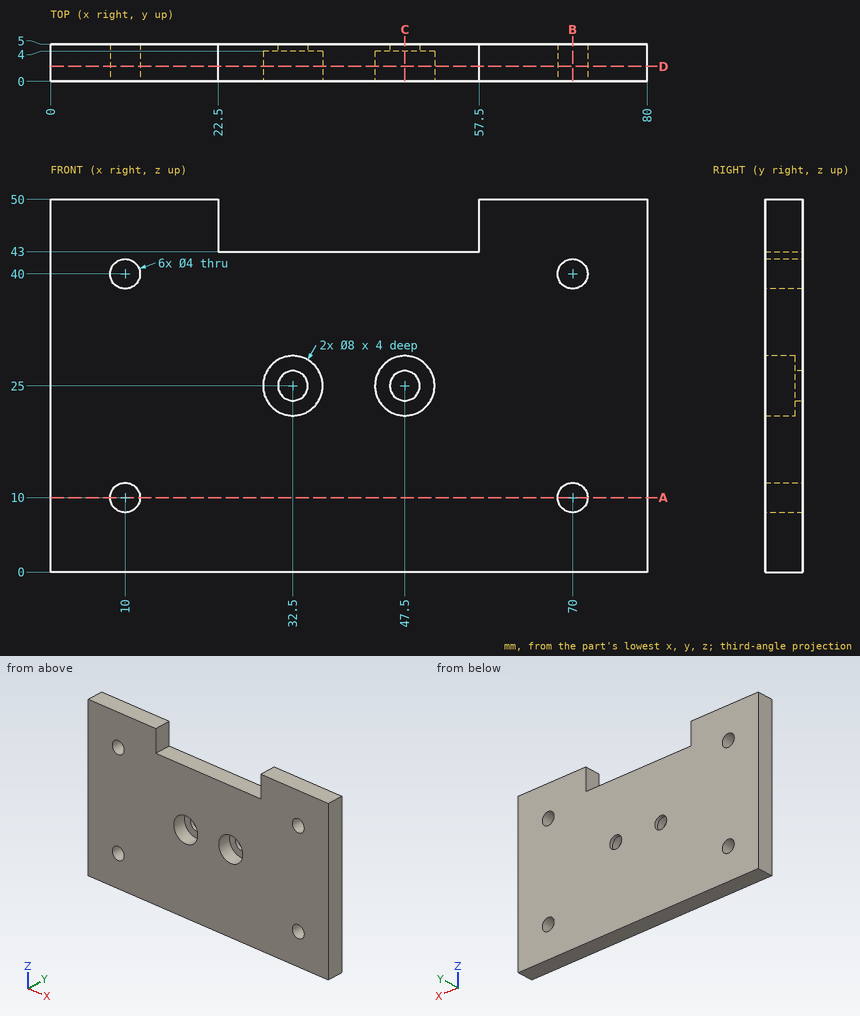
Verification items for this drawing (mm, ordinates from the low corner). Round coordinates to 2 decimals unless told otherwise and drop trailing zeros. Write each loop counter-clockwise with the first axis right and the second up, starting at its lowest first coordinate (ties: lowest second). Pieces come first, ordered by that corner, then holes. Notation, with made-up numbers: (-6, -25) - (15, -25) arc R38 cw to (15, 14) - close; hole circle Ø9 at (31.25, 50). An arc over 180 degrees is marked (long way). Answer as a JSON object with one key per item and string values. Group by question number.
Q1. Thickness scan on line 1 (X direction, y = 4.55, z = 25); line 2 (X direction, y = 3.65, z = 10); line 3 (Z direction, x = 70, y = 1.2). Record the ranges inside material, lowest first.
Q2. Section check B-B, the plane x = 70. Enter the section's corners in (y, z).
Q3. Go/stop test with flat-tipped pins: pin 1 Ø2.5 at (x, z) = (47, 26) entering from -Y; pin 2 Ø1.5 at (x, y) = (47.5, 1) entering from +Z. Record where each tip stops, or that it passes through.
Q4. Section check A-A, the plane z = 10. Enter the section's corners in (x, y), plus the area to 3 significant figures.
Q5. Section check C-C, the plane x = 47.5. Enter the section's corners in (y, z).
Q6. Section check D-D, the plane y = 2. Enter the section's corners in (x, z).
Found:
{
 "1": {"line 1": "x = 0 to 30.5, 34.5 to 45.5, 49.5 to 80", "line 2": "x = 0 to 8, 12 to 68, 72 to 80", "line 3": "z = 0 to 8, 12 to 38, 42 to 50"},
 "2": {"outline": "(0, 0) - (5, 0) - (5, 8) - (0, 8) - close; (0, 12) - (5, 12) - (5, 38) - (0, 38) - close; (0, 42) - (5, 42) - (5, 50) - (0, 50) - close"},
 "3": {"pin 1": "stops at y = 4", "pin 2": "stops at z = 43"},
 "4": {"outline": "(0, 0) - (8, 0) - (8, 5) - (0, 5) - close; (12, 0) - (68, 0) - (68, 5) - (12, 5) - close; (72, 0) - (80, 0) - (80, 5) - (72, 5) - close", "area": "360 mm^2"},
 "5": {"outline": "(0, 0) - (5, 0) - (5, 23) - (4, 23) - (4, 21) - (0, 21) - close; (0, 29) - (4, 29) - (4, 27) - (5, 27) - (5, 43) - (0, 43) - close"},
 "6": {"outline": "(0, 0) - (80, 0) - (80, 50) - (57.5, 50) - (57.5, 43) - (22.5, 43) - (22.5, 50) - (0, 50) - close; hole circle Ø4 at (10, 10); hole circle Ø4 at (10, 40); hole circle Ø8 at (32.5, 25); hole circle Ø8 at (47.5, 25); hole circle Ø4 at (70, 10); hole circle Ø4 at (70, 40)"}
}
